```python
from build123d import *

# Parameters (mm, degrees)
BOSS_EXTRUDE1_DEPTH = 891.7


with BuildPart() as part:
    # Sketch1 → Boss-Extrude1 (new body)
    with BuildSketch(Plane.XY):
        with BuildLine():
            Line((21.307457755, 0), (-12.692542245, 0))
            Line((-12.692542245, 0), (-12.692542245, 4))
            Line((-12.692542245, 4), (-3.192542245, 4))
            Line((-3.192542245, 4), (-3.192542245, 9.8))
            Line((-3.192542245, 9.8), (0.390557455, 9.8))
            Line((0.390557455, 9.8), (1.307457755, 15))
            ThreePointArc((1.307457755, 15), (4.307457755, 26.196152423), (7.307457755, 15))
            Line((7.307457755, 15), (8.224358055, 9.8))
            Line((8.224358055, 9.8), (11.807457755, 9.8))
            Line((11.807457755, 9.8), (11.807457755, 4))
            Line((11.807457755, 4), (21.307457755, 4))
            Line((21.307457755, 4), (21.307457755, 0))
        make_face()
    extrude(amount=BOSS_EXTRUDE1_DEPTH)


solid = part.part
```
Geometry check sheet. Reference: the model listing, model coordinates, mm. Give positions to 0.01 mm unless a question says otherwise; leave off trailing zeros. Write each loop counter-clockwise with the first axis right and the second up, starting at its lowest first coordinate (ties: lowest second). Pieces come first, ordered by that corner, then holes.
1) Material ranges on L1, parallel to X at y = 14.25, z = 790; L2, parallel to Y at x = -8.5, z = 621; L3, parallel to X at y = 6.5, z = 733, recorded low to high.
2) Gauge pin test, flat ends, axial feed: pin 1 (3 mm diameter, centred on y = 6, z = 236, fed in from -X); pin 2 (1.1 mm diameter, centred on x = 11, z = 614.5, fed in from +Y); pin 3 (4.5 mm diameter, centred on y = 7, z = 530, fed in from +X); pin 4 (6.5 mm diameter, centred on y = 7, z = 631.5, fed in from -X). Record the tip position at first contact, or that the pin passes through.
3) Section check B-B, the plane y = 20.75. Record the boundary of the cut face in (x, z).
4) Section check A-A, the plane z = 57. Record the boundary of the cut face in (x, y).
Computed:
1. L1: x = 1.18 to 7.44
1. L2: y = 0 to 4
1. L3: x = -3.19 to 11.81
2. pin 1: stops at x = -3.19
2. pin 2: stops at y = 9.8
2. pin 3: stops at x = 11.81
2. pin 4: stops at x = -12.69
3. outline: (-1.67, 0) - (10.28, 0) - (10.28, 891.7) - (-1.67, 891.7) - close
4. outline: (-12.69, 0) - (21.31, 0) - (21.31, 4) - (11.81, 4) - (11.81, 9.8) - (8.22, 9.8) - (7.31, 15) arc R6 ccw (long way) to (1.31, 15) - (0.39, 9.8) - (-3.19, 9.8) - (-3.19, 4) - (-12.69, 4) - close
